```python
from build123d import *

# Parameters (mm, degrees)
SKETCH1_W           = 63.5
SKETCH1_H           = 63.5
BOSS_EXTRUDE1_DEPTH = 1.5875
FILLET1_R           = 0.508
FILLET2_R           = 3.175


with BuildPart() as part:
    # Sketch1 → Boss-Extrude1 (new body)
    with BuildSketch(Plane(origin=(0, 0, 0), x_dir=(1, 0, 0), z_dir=(0, 1, 0))):
        with Locations((31.75, 31.75)):
            Rectangle(SKETCH1_W, SKETCH1_H)
        with BuildLine():
            Line((24.384, 42.111215435), (24.384, 39.116))
            Line((24.384, 39.116), (21.388784565, 39.116))
            ThreePointArc((21.388784565, 39.116), (31.75, 19.0373), (42.111215435, 39.116))
            Line((42.111215435, 39.116), (39.116, 39.116))
            Line((39.116, 39.116), (39.116, 42.111215435))
            ThreePointArc((39.116, 42.111215435), (31.75, 44.4627), (24.384, 42.111215435))
        make_face(mode=Mode.SUBTRACT)
    extrude(amount=BOSS_EXTRUDE1_DEPTH)

    # Fillet1
    fillet1_edges = [part.edges().sort_by_distance(p)[0] for p in [
        (24.384, 0.79375, -39.116),
        (39.116, 0.79375, -39.116),
    ]]
    fillet(fillet1_edges, radius=FILLET1_R)

    # Fillet2
    fillet2_edges = [part.edges().sort_by_distance(p)[0] for p in [
        (0, 0.79375, -63.5),
        (63.5, 0.79375, -63.5),
        (63.5, 0.79375, 0),
        (0, 0.79375, 0),
    ]]
    fillet(fillet2_edges, radius=FILLET2_R)


solid = part.part
```
Read the model definition and answer for the solid it produces. Units are mm, in the model's axes. A direction names the side the tool comes from. Coordinates: 2 decimals unless noted, no trailing zeros. Order: outer loops, then holes, each group sorted by start corner. A loop starts at its lowest first (then second) coordinate and runs counter-clockwise, first axis right, second up. Notation, with made-up numbers: (-22, -4) - (-5, -4) arc R28 ccw to (-5, 31) - close; hole circle Ø1 at (75, 84). An arc over 180 degrees is marked (long way). Answer as a JSON object with one key per item and string values. Group by question number.
Item 1: Consider probe 1 along X at (y, z) = (1.1, -31.75); probe 2 along Z at (x, y) = (38.5, 0.45); probe 3 along Z at (x, y) = (24, 1). Determine where each line is inside the solid, lowest interval first. Write a range as from..to.
Item 2: Section C-C (y = 1.25) is taken. Give the vertices of the cut face in (x, z) (3 decimals).
Item 3: Section A-A (z = -31.75) is taken. Give the vertices of the cut face in (x, y), plus the area to 3 significant figures.
Item 4: The mould has two halves that part along Z. Classify faces 3 (the face through (0, 1, -31)), 4 (the face through (39.116, 1, -41)), 5 (the face through (31, 1, 0)): +Z half, -Z half, draft (parallel to the pull), parting line (faces both ways), or undercut.
Item 5: A tool of negligible diameter and unlimited length cuts with its end or side. For faces 1 (the face through (17, 0, -32)), 2 (the face through (31.86, 0.783, -44.462)), from which of +Z, -Z, +X, -X, +Y, -Y can it reach the whole face along a straight path? Write none if from no direction.
Item 6: Section B-B (x = 31.75) is taken. Give the vertices of the cut face in (y, z).
Results are:
{
 "1": {"probe 1": "x = 0..19.04, 44.46..63.5", "probe 2": "z = -63.5..-42.52, -20.98..0", "probe 3": "z = -63.5..-39.13, -21.67..0"},
 "2": {"outline": "(0, -60.325) arc R3.175 ccw to (3.175, -63.5) - (60.325, -63.5) arc R3.175 ccw to (63.5, -60.325) - (63.5, -3.175) arc R3.175 ccw to (60.325, 0) - (3.175, 0) arc R3.175 ccw to (0, -3.175) - close; hole (21.389, -39.116) - (23.876, -39.116) arc R0.508 cw to (24.384, -39.624) - (24.384, -42.111) arc R12.713 ccw to (39.116, -42.111) - (39.116, -39.624) arc R0.508 cw to (39.624, -39.116) - (42.111, -39.116) arc R12.713 ccw (long way) to start"},
 "3": {"outline": "(0, 0) - (19.04, 0) - (19.04, 1.59) - (0, 1.59) - close; (44.46, 0) - (63.5, 0) - (63.5, 1.59) - (44.46, 1.59) - close", "area": "60.4 mm^2"},
 "4": {"face 3": "draft", "face 4": "undercut", "face 5": "+Z half"},
 "5": {"face 1": "+Z, -Z, +X, -X, -Y", "face 2": "+Y, -Y"},
 "6": {"outline": "(0, -63.5) - (1.59, -63.5) - (1.59, -44.46) - (0, -44.46) - close; (0, -19.04) - (1.59, -19.04) - (1.59, 0) - (0, 0) - close"}
}
